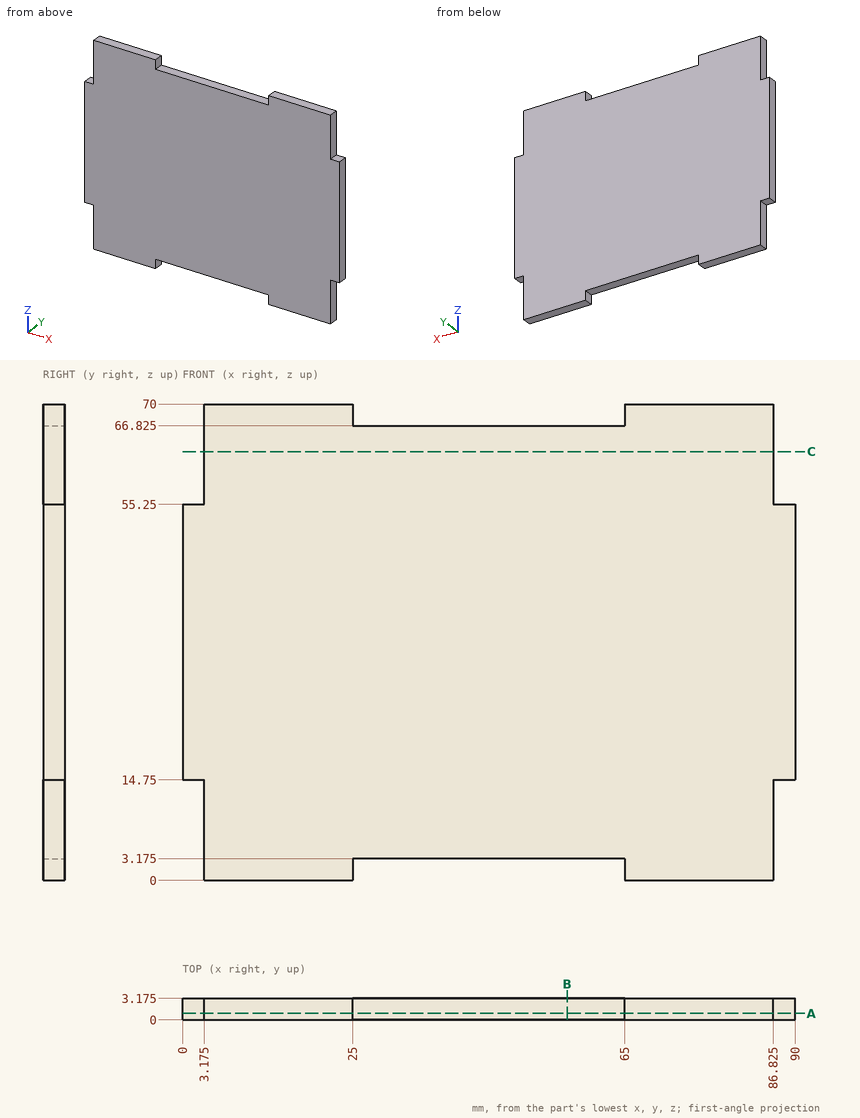
Verification items for this drawing (mm, ordinates from the low corner). Round coordinates to 2 decimals unless told otherwise and drop trailing zeros. Order: outer loops, then holes, each group sorted by start corner. A loop starts at its lowest first (then second) coordinate and runs counter-clockwise, first axis right, second up. Notation, with made-up numbers: (-8, -2) - (38, -2) arc R25 ccw to (38, 33) - close; hole circle Ø11 at (7.5, 89). An arc over 180 degrees is marked (long way). Use CSV: the item, a comma, the result in double quotes. Start each with the question number.
1) Thickness scan on L1, parallel to X at y = 0.9, z = 67 (3 decimals); L2, parallel to Z at x = 31, y = 1 (3 decimals); L3, parallel to X at y = 2.65, z = 65.5 (3 decimals). Record the ranges inside material, lowest first.
2) Go/stop test with flat-tipped pins: P1, Ø1.6, axis at y = 1.5, z = 68, coming from the -X side (3 decimals); P2, Ø1.5, axis at x = 49.5, y = 2.5, coming from the +Z side (3 decimals); P3, Ø1.6, axis at y = 2, z = 1, coming from the +X side (3 decimals). Record where each tip stops, or that it passes through.
3) Section check C-C, the plane z = 63. Record the cut outline in (x, y) (3 decimals), plus the area to 3 significant figures.
4) Section check B-B, the plane x = 56.5. Record the cut outline in (y, z) (3 decimals), plus the area to 3 significant figures.
5) Section check A-A, the plane y = 0.95. Record the cut outline in (x, z) (3 decimals).
Answers:
1,L1,"x = 3.175 to 25, 65 to 86.825"
1,L2,"z = 3.175 to 66.825"
1,L3,"x = 3.175 to 86.825"
2,P1,"stops at x = 3.175"
2,P2,"stops at z = 66.825"
2,P3,"stops at x = 86.825"
3,outline,"(3.175, 0) - (86.825, 0) - (86.825, 3.175) - (3.175, 3.175) - close"
3,area,"266 mm²"
4,outline,"(0, 3.175) - (3.175, 3.175) - (3.175, 66.825) - (0, 66.825) - close"
4,area,"202 mm²"
5,outline,"(0, 14.75) - (3.175, 14.75) - (3.175, 0) - (25, 0) - (25, 3.175) - (65, 3.175) - (65, 0) - (86.825, 0) - (86.825, 14.75) - (90, 14.75) - (90, 55.25) - (86.825, 55.25) - (86.825, 70) - (65, 70) - (65, 66.825) - (25, 66.825) - (25, 70) - (3.175, 70) - (3.175, 55.25) - (0, 55.25) - close"
